The listing builds one solid part. Answer for the finished solid, in the listing's coordinates (mm). A direction names the side the tool comes from. Round coordinates to 2 decimals unless told otherwise and drop trailing zeros. Order: outer loops, then holes, each group sorted by start corner. A loop starts at its lowest first (then second) coordinate and runs counter-clockwise, first axis right, second up. Notation, with made-up numbers: (20.25, 30) - (24.25, 30) arc R15 cw to (24.25, 41) - close; hole circle Ø6 at (22.25, 16). An arc over 180 degrees is marked (long way). One line per item, written item: value. Start each with the question number.
1. Section B-B, the plane y = 3.35 is taken. Give the vertices of the cut face in (x, z) (3 decimals), then the cut area to 3 significant figures.
2. Section C-C, the plane z = -1.5 is taken. Give the vertices of the cut face in (x, y) (1 decimal), then the cut area to 3 significant figures.
3. A tool of negligible diameter and unlimited length cuts with its end or side. For faces 1 (the flat face through (15, 1.58, 0)), 2 (the flat face through (-28, 4.04, 0)), 3 (the cylindrical face through (-0.207, 3.256, 0.52)), from which of +Z, -Z, +X, -X, +Y, -Y can it reach the whole face along a straight path? Write none if from no direction.
4. Straight lines are drawn through the part: line 1 (X direction, y = 0.5, z = 2) (3 decimals); line 2 (X direction, y = 1.05, z = 0.5) (3 decimals); line 3 (X direction, y = 2.7, z = 0.25) (3 decimals). For each, find the intervals that lie inside material, in ascending order.
5. Section A-A, the plane x = 27.97 is taken. Give the vertices of the cut face in (y, z) (3 decimals), then the cut area to 3 significant figures.
6. For a pull along X with two mould halves and no side action, classify faces 4 (the cylindrical face through (29.17, 0.41, 1.88)), 5 (the flat face through (-3, 4.3, 0)), 6 (the flat face through (-30.075, 2, 0)) as released by +X, released by -X, zero draft, split by the parting line, or undercut.
7. Flat-ended cylindrical pins translate along their axes: P1, Ø1, axis at x = 10.5, z = 1.5, coming from the +Y side; P2, Ø0.8, axis at x = 14.5, y = 1.5, coming from the -Z side; P3, Ø1, axis at x = -9.5, z = 0, coming from the -Y side; P4, Ø4, axis at x = 12, z = -2.5, coming from the +Y side. Find the tip coordinate at first contact, or state that the pin passes through.
8. Section D-D, the plane x = -2.55 is taken. Give the vertices of the cut face in (y, z) (3 decimals), then the cut area to 3 significant figures.
from build123d import *

# Parameters (mm, degrees)
SKETCH1_W            = 60.15
SKETCH1_H            = 8
BOSS_EXTRUDE1_DEPTH  = 0.83
SKETCH2_W            = 6.45
SKETCH2_H            = 6.45
SKETCH2_R            = 2.4
BOSS_EXTRUDE2_DEPTH  = 1.41
SKETCH2_3_R          = 2.4
BOSS_EXTRUDE3_DEPTH  = 3.47
SKETCH3_W            = 4.2
SKETCH3_H            = 8
BOSS_EXTRUDE4_DEPTH  = 3.21
M2_CLEARANCE_HOLE1_D = 2.4
SKETCH6_W            = 5
SKETCH6_H            = 5
BOSS_EXTRUDE5_DEPTH  = 0.75


with BuildPart() as part:
    # Sketch1 → Boss-Extrude1 (new body)
    with BuildSketch(Plane(origin=(0, 0, 0), x_dir=(1, 0, 0), z_dir=(0, 1, 0))):
        Rectangle(SKETCH1_W, SKETCH1_H)
    extrude(amount=BOSS_EXTRUDE1_DEPTH)

    # Sketch2 → Boss-Extrude2 (add)
    # profile 1 of 2: a face of its own
    with BuildSketch(Plane(origin=(0, 0.83, 0), x_dir=(1, 0, 0), z_dir=(0, 1, 0))):
        with Locations((-2.55, 0)):
            Rectangle(SKETCH2_W, SKETCH2_H)
        with Locations((-2.55, 0)):
            Circle(SKETCH2_R, mode=Mode.SUBTRACT)
    # profile 2 of 2: a face of its own
    with BuildSketch(Plane(origin=(0, 0.83, 0), x_dir=(1, 0, 0), z_dir=(0, 1, 0))):
        with Locations((-2.55, 0)):
            Circle(SKETCH2_R)
    extrude(amount=BOSS_EXTRUDE2_DEPTH)

    # Sketch2<3> → Boss-Extrude3 (add)
    with BuildSketch(Plane(origin=(0, 0.83, 0), x_dir=(1, 0, 0), z_dir=(0, 1, 0))):
        with Locations(Location((-2.55, 0, 0), (0, 0, 90))):
            Circle(SKETCH2_3_R)
    extrude(amount=BOSS_EXTRUDE3_DEPTH)

    # Sketch3 → Boss-Extrude4 (add)
    with BuildSketch(Plane(origin=(0, 0.83, 0), x_dir=(1, 0, 0), z_dir=(0, 1, 0))):
        with Locations((-27.975, 0)):
            Rectangle(SKETCH3_W, SKETCH3_H)
    extrude(amount=BOSS_EXTRUDE4_DEPTH)

    # M2 Clearance Hole1 (through all)
    with Locations(Plane(origin=(0, 0.83, 0), x_dir=(1, 0, 0), z_dir=(0, 1, 0))):
        with Locations((24.52, 2.065), (27.97, 2.065), (27.97, -1.935), (-23.39, -1.925), (-22.33, -2.005)):
            Hole(M2_CLEARANCE_HOLE1_D / 2)

    # Sketch6 → Boss-Extrude5 (add)
    with BuildSketch(Plane(origin=(0, 0.83, 0), x_dir=(1, 0, 0), z_dir=(0, 1, 0))):
        with Locations((15.475, 0)):
            Rectangle(SKETCH6_W, SKETCH6_H)
    extrude(amount=BOSS_EXTRUDE5_DEPTH)


solid = part.part
Answer list:
1. outline: (-30.075, -4) - (-25.875, -4) - (-25.875, 4) - (-30.075, 4) - close; circle Ø4.8 at (-2.55, 0)
1. area: 51.7 mm²
2. outline: (-30.1, 0) - (23.5, 0) - (23.5, 0.8) - (18, 0.8) - (18, 1.6) - (13, 1.6) - (13, 0.8) - (0.7, 0.8) - (0.7, 2.2) - (-0.7, 2.2) - (-0.7, 4.3) - (-4.4, 4.3) - (-4.4, 2.2) - (-5.8, 2.2) - (-5.8, 0.8) - (-25.9, 0.8) - (-25.9, 4) - (-30.1, 4) - close; (25.6, 0) - (26.9, 0) - (26.9, 0.8) - (25.6, 0.8) - close; (29, 0) - (30.1, 0) - (30.1, 0.8) - (29, 0.8) - close
2. area: 80.5 mm²
3. face 1: +Z, -Z, +X, +Y
3. face 2: +Z, -Z, -X, +Y
3. face 3: +Y
4. line 1: x = -30.075 to -24.588, -21.13 to 26.772, 29.168 to 30.075
4. line 2: x = -30.075 to -25.875, -5.775 to 0.675, 12.975 to 17.975
4. line 3: x = -30.075 to -25.875, -4.937 to -0.163
5. outline: (0, -4) - (0.83, -4) - (0.83, -3.265) - (0, -3.265) - close; (0, -0.865) - (0.83, -0.865) - (0.83, 0.735) - (0, 0.735) - close; (0, 3.135) - (0.83, 3.135) - (0.83, 4) - (0, 4) - close
5. area: 2.66 mm²
6. face 4: undercut
6. face 5: zero draft
6. face 6: released by -X
7. P1: stops at y = 0.83
7. P2: stops at z = -2.5
7. P3: stops at y = 0
7. P4: stops at y = 1.58
8. outline: (0, -4) - (0.83, -4) - (0.83, -3.225) - (2.24, -3.225) - (2.24, -2.4) - (4.3, -2.4) - (4.3, 2.4) - (2.24, 2.4) - (2.24, 3.225) - (0.83, 3.225) - (0.83, 4) - (0, 4) - close
8. area: 25.6 mm²
